Can you work these out from the model? Positions are in its coordinate system, mm. A direction names the side the tool comes from. Round coordinates to 2 decimals unless told otherwise and drop trailing zeros. Order: outer loops, then holes, each group sorted by start corner. A loop starts at its lowest first (then second) coordinate and runs counter-clockwise, first axis right, second up. Notation, with made-up numbers: (61.25, -3.75) -> (65.25, -3.75) arc R19 ccw to (65.25, 31.25) -> close; hole circle Ø11 at (-4, 3.5). An arc over 180 degrees is marked (long way). Use a Markdown table: item, result. Add a question column.
Q1. For faces 1 (the face through (8.24, 14.27, 1.48)), 2 (the face through (-22.01, 22.04, -7.6)), which set-ups out of +Z, -Z, +X, -X, +Y, -Y let a thin tool reach every point of the face, with its end or its side?
Q2. If we section it at A-A on y = 32.5: List the corners of the cut face in (x, z) for me, plus the area to 3 significant figures.
Q3. I'm going to push flat-ended pins straight in: pin 1 Ø1.5 at (x, y) = (-33, 0.5) entering from -Z; pin 2 Ø0.5 at (x, y) = (21.5, 21.5) entering from -Z; pin 3 Ø1 at (x, z) = (-4, -0.5) entering from -Y; pin 4 Ø9 at (x, y) = (0, 0) entering from -Z. Where does each tip first touch, or does it pass through?
Q4. If we section it at B-B on z = -9.25: List the corners of the cut face in (x, y) for me.
Q5. I need wall thicknesses on line 1 along Y through (x, z) = (0, 1.05); line 2 along Y through (x, z) = (0, -7.5). Which ranges of each line are inside material? Lowest first, please. Write a range as [from, to].
```python
from build123d import *

# Parameters (mm, degrees)
SKETCH_2_R          = 35
SKETCH_2_R_2        = 5.5
EXTRUDE_1_DEPTH     = 5
EXTRUDE_START       = 15
SKETCH_3_R          = 35
SKETCH_3_R_2        = 30.1
EXTRUDE_2_DEPTH     = 15
SKETCH_4_R          = 1.55
CUT_EXTRUDE_1_DEPTH = 10
CUT_EXTRUDE_5_DEPTH = 15
FILLET_1_R          = 1
CUT_EXTRUDE_START   = -2
SKETCH_10_R         = 35
CUT_EXTRUDE_6_DEPTH = 2
CUT_EXTRUDE_7_DEPTH = 10


with BuildPart() as part:
    # 草图2 → 凸台-拉伸1 (new body)
    with BuildSketch(Plane.XY):
        Circle(SKETCH_2_R)
        Circle(SKETCH_2_R_2, mode=Mode.SUBTRACT)
    extrude(amount=EXTRUDE_1_DEPTH)

    # 草图3 → 凸台-拉伸2 (add)
    with BuildSketch(Plane(origin=(0, 0, 0), x_dir=(-1, 0, 0), z_dir=(0, 0, -1)).offset(EXTRUDE_START)):
        Circle(SKETCH_3_R)
        Circle(SKETCH_3_R_2, mode=Mode.SUBTRACT)
    extrude(amount=-EXTRUDE_2_DEPTH)

    # 草图4 → 切除-拉伸1 (cut)
    with BuildSketch(Plane(origin=(0, 0, -15), x_dir=(-1, 0, 0), z_dir=(0, 0, -1))):
        with Locations((0, 32.5)):
            Circle(SKETCH_4_R)
        with Locations((32.5, 0)):
            Circle(SKETCH_4_R)
        with Locations((0, -32.5)):
            Circle(SKETCH_4_R)
        with Locations((-32.5, 0)):
            Circle(SKETCH_4_R)
    extrude(amount=-CUT_EXTRUDE_1_DEPTH, mode=Mode.SUBTRACT)

    # 草图9 → 切除-拉伸5 (cut)
    with BuildSketch(Plane(origin=(0, 0, -15), x_dir=(-1, 0, 0), z_dir=(0, 0, -1))):
        with BuildLine():
            ThreePointArc((-22.013313369, 20.528615017), (-22.026376234, 22.026376234), (-20.528615017, 22.013313369))
            ThreePointArc((-20.528615017, 22.013313369), (-21.283914114, 21.283914114), (-22.013313369, 20.528615017))
        make_face()
        with BuildLine():
            ThreePointArc((20.528615017, 22.013313369), (22.026376234, 22.026376234), (22.013313369, 20.528615017))
            ThreePointArc((22.013313369, 20.528615017), (21.283914114, 21.283914114), (20.528615017, 22.013313369))
        make_face()
        with BuildLine():
            ThreePointArc((22.013313369, -20.528615017), (22.026376234, -22.026376234), (20.528615017, -22.013313369))
            ThreePointArc((20.528615017, -22.013313369), (21.283914114, -21.283914114), (22.013313369, -20.528615017))
        make_face()
        with BuildLine():
            ThreePointArc((-20.528615017, -22.013313369), (-22.026376234, -22.026376234), (-22.013313369, -20.528615017))
            ThreePointArc((-22.013313369, -20.528615017), (-21.283914114, -21.283914114), (-20.528615017, -22.013313369))
        make_face()
    extrude(amount=-CUT_EXTRUDE_5_DEPTH, mode=Mode.SUBTRACT)

    # 圆角1
    # the kernel refuses this fillet: 1 mm, written as the material it takes off along each edge
    with BuildSketch(Plane(origin=(0, 0, -15), x_dir=(-0.7403558797037455, 0.6722151228498904, 0), z_dir=(-0.6722151228498904, -0.7403558797037455, 0))) as fillet_1_piece_1:
        with BuildLine():
            CenterArc((30.1 + FILLET_1_R, -FILLET_1_R), FILLET_1_R, 90, 90)
            Line((30.1, -FILLET_1_R), (30.1, 0))
            Line((30.1, 0), (30.1 + FILLET_1_R, 0))
        make_face()
    revolve(axis=Axis((0, 0, -15), (0, 0, -1)), revolution_arc=95.523479776, mode=Mode.SUBTRACT)
    with BuildSketch(Plane(origin=(0, 0, -15), x_dir=(0.6722151228498918, 0.7403558797037441, 0), z_dir=(-0.7403558797037441, 0.6722151228498918, 0))) as fillet_1_piece_2:
        with BuildLine():
            CenterArc((30.1 + FILLET_1_R, -FILLET_1_R), FILLET_1_R, 90, 90)
            Line((30.1, -FILLET_1_R), (30.1, 0))
            Line((30.1, 0), (30.1 + FILLET_1_R, 0))
        make_face()
    revolve(axis=Axis((0, 0, -15), (0, 0, -1)), revolution_arc=95.523479776, mode=Mode.SUBTRACT)
    with BuildSketch(Plane(origin=(0, 0, -15), x_dir=(0.7403558797037453, -0.6722151228498905, 0), z_dir=(0.6722151228498905, 0.7403558797037453, 0))) as fillet_1_piece_3:
        with BuildLine():
            CenterArc((30.1 + FILLET_1_R, -FILLET_1_R), FILLET_1_R, 90, 90)
            Line((30.1, -FILLET_1_R), (30.1, 0))
            Line((30.1, 0), (30.1 + FILLET_1_R, 0))
        make_face()
    revolve(axis=Axis((0, 0, -15), (0, 0, -1)), revolution_arc=95.523479776, mode=Mode.SUBTRACT)
    with BuildSketch(Plane(origin=(0, 0, -15), x_dir=(-1, 0, 0), z_dir=(0, -1, 0))) as fillet_1_piece_4:
        with BuildLine():
            CenterArc((30.1 + FILLET_1_R, -FILLET_1_R), FILLET_1_R, 90, 90)
            Line((30.1, -FILLET_1_R), (30.1, 0))
            Line((30.1, 0), (30.1 + FILLET_1_R, 0))
        make_face()
    revolve(axis=Axis((0, 0, -15), (0, 0, -1)), revolution_arc=47.760430641, mode=Mode.SUBTRACT)
    with BuildSketch(Plane(origin=(0, 0, -15), x_dir=(-0.6722320403041436, -0.7403405189428228, 0), z_dir=(0.7403405189428228, -0.6722320403041436, 0))) as fillet_1_piece_5:
        with BuildLine():
            CenterArc((30.1 + FILLET_1_R, -FILLET_1_R), FILLET_1_R, 90, 90)
            Line((30.1, -FILLET_1_R), (30.1, 0))
            Line((30.1, 0), (30.1 + FILLET_1_R, 0))
        make_face()
    revolve(axis=Axis((0, 0, -15), (0, 0, -1)), revolution_arc=47.760430641, mode=Mode.SUBTRACT)

    # 草图10 → 切除-拉伸6 (cut)
    with BuildSketch(Plane.XY.offset(5).offset(CUT_EXTRUDE_START)):
        with Locations(Location((0, 0, 0), (0, 0, 180))):
            Circle(SKETCH_10_R)
    extrude(amount=CUT_EXTRUDE_6_DEPTH, mode=Mode.SUBTRACT)

    # 草图11 → 切除-拉伸7 (cut)
    with BuildSketch(Plane(origin=(0, 0, 0), x_dir=(-1, 0, 0), z_dir=(0, 0, -1))):
        with BuildLine():
            Line((12.990381057, 7.5), (15.588457268, 9))
            ThreePointArc((15.588457268, 9), (18, 0), (15.588457268, -9))
            Line((15.588457268, -9), (12.990381057, -7.5))
            ThreePointArc((12.990381057, -7.5), (15, 0), (12.990381057, 7.5))
        make_face()
        with BuildLine():
            Line((-7.5, 12.990381057), (-9, 15.588457268))
            ThreePointArc((-9, 15.588457268), (0, 18), (9, 15.588457268))
            Line((9, 15.588457268), (7.5, 12.990381057))
            ThreePointArc((7.5, 12.990381057), (0, 15), (-7.5, 12.990381057))
        make_face()
        with BuildLine():
            Line((7.5, -12.990381057), (9, -15.588457268))
            ThreePointArc((9, -15.588457268), (0, -18), (-9, -15.588457268))
            Line((-9, -15.588457268), (-7.5, -12.990381057))
            ThreePointArc((-7.5, -12.990381057), (0, -15), (7.5, -12.990381057))
        make_face()
        with BuildLine():
            Line((-12.990381057, -7.5), (-15.588457268, -9))
            ThreePointArc((-15.588457268, -9), (-18, 0), (-15.588457268, 9))
            Line((-15.588457268, 9), (-12.990381057, 7.5))
            ThreePointArc((-12.990381057, 7.5), (-15, 0), (-12.990381057, -7.5))
        make_face()
    extrude(amount=-CUT_EXTRUDE_7_DEPTH, mode=Mode.SUBTRACT)


solid = part.part
```
Answer below:
| question | item | result |
|---|---|---|
| 1 | face 1 | +Z, -Z |
| 1 | face 2 | -Z |
| 2 | outline | (-12.99, -15) -> (-1.55, -15) -> (-1.55, -5) -> (1.55, -5) -> (1.55, -15) -> (12.99, -15) -> (12.99, 3) -> (-12.99, 3) -> close |
| 2 | area | 437 mm² |
| 3 | pin 1 | z = -5 |
| 3 | pin 2 | z = 0 |
| 3 | pin 3 | y = -34.82 |
| 3 | pin 4 | through |
| 4 | outline | circle Ø70 at (0, 0); hole circle Ø3.1 at (-32.5, 0); hole (-22.01, -20.53) arc R1.05 ccw (long way) to (-20.53, -22.01) arc R30.1 ccw to (20.53, -22.01) arc R1.05 ccw (long way) to (22.01, -20.53) arc R30.1 ccw to (22.01, 20.53) arc R1.05 ccw (long way) to (20.53, 22.01) arc R30.1 ccw to (-20.53, 22.01) arc R1.05 ccw (long way) to (-22.01, 20.53) arc R30.1 ccw to start; hole circle Ø3.1 at (0, -32.5); hole circle Ø3.1 at (0, 32.5); hole circle Ø3.1 at (32.5, 0) |
| 5 | line 1 | [-35, -18], [-15, -5.5], [5.5, 15], [18, 35] |
| 5 | line 2 | [-35, -34.05], [-30.95, -30.1], [30.1, 30.95], [34.05, 35] |
